Part model, mm, in its own coordinate system. A direction names the side the tool comes from. Give positions to 0.01 mm unless a question says otherwise; leave off trailing zeros. Write each loop counter-clockwise with the first axis right and the second up, starting at its lowest first coordinate (ties: lowest second). Pieces come first, ordered by that corner, then holes. Notation, with made-up numbers: M 43,28 L 58,28 A28 cw 58,63 Z; hole C 78,49.5 d5. An arc over 180 degrees is marked long. Write item = value, one per line. Start each with the question number.
Autodesk Inventor part; units mm, degrees
ref_plane "YZ Plane" through (0, 0, 0) normal (1, 0, 0) x (0, 1, 0)
ref_plane "XZ Plane" through (0, 0, 0) normal (0, 1, 0) x (-1, 0, 0)
ref_plane "XY Plane" through (0, 0, 0) normal (0, 0, 1) x (1, 0, 0)
sketch "Sketch1" plane through (0, 0, 0) normal (1, 0, 0) x (0, 1, 0)
  line L0 (0, 280.159) -> (0, -280.159)
  line L1 (0, 15) -> (100, 15)
  line L2 (100, 15) -> (100, 15)
  line L3 (105, 20) -> (125, 20)
  line L4 (130, 15) -> (130, -15)
  line L5 (125, -20) -> (105, -20)
  line L6 (100, -15) -> (100, -15)
  line L7 (100, -15) -> (0, -15)
  line L8 (0, 15) -> (0, -15)
  line L9 (0, 0) -> (130, 0)
  arc A0 (128, -20) -> (130, -18) centre (128, -18) ccw
  arc A1 (125, -20) -> (130, -15) centre (125, -15) ccw
  arc A2 (130, 15) -> (125, 20) centre (125, 15) ccw
  arc A3 (105, 20) -> (100, 15) centre (105, 15) ccw
  arc A4 (100, -15) -> (105, -20) centre (105, -15) ccw
  line L10 (10, 15) -> (10, -15)
  point P0 (130, 20)
  point P1 (130, -20)
  point P2 (100, -20)
  dimension "d0" = 560.3179
  dimension "d1" = 40
  dimension "d2" = 30
  dimension "d3" = 30
  dimension "d4" = 260
  dimension "d5" = 2
  dimension "d6" = 5
  dimension "d7" = 20
revolve "Revolution1" add sketch "Sketch1" angle 360 about axis through (0, 0, 280.159) along (0, 0, -1) contours L1 A3 L3 A2 L4 L9 L10 | L9 L4 A1 L5 A4 L7 L10
properties part number "wiel"
Q1. Slice it at C-C (z = -4.5). Give the cut face in (x, y), and give its area (3 significant figures).
Q2. Probe line 1 along X through (y, z) = (0, 8); line 2 along Z through (x, y) = (-35, -89); line 3 along Z through (x, y) = (-107, 65). List the from-to ranges inside material, lowest first.
Q3. Tool access for faces 1 (the face through (102, -28, -20)), 2 (the face through (-21, -1, 15)), 3 (the face through (-21, -1, -15)): list every direction of +Z, -Z, +X, -X, +Y, -Y with a clear straight run to the whole face (end or side of a thin tool).
Q4. Drop flat-ended pins along their axis: P1, Ø8, axis at x = 73, y = 0, coming from the +Z side; P2, Ø5, axis at x = 8.5, z = 7, coming from the -Y side; P3, Ø1, axis at y = 52, z = 9.5, coming from the -X side. Give the stop position or say it passes through.
Q5. Two-plate mould, pull along X, no slides. Class faces 4 (the face through (-9.76, -2.17, -0.21)), 5 (the face through (39.048, 123.997, -0.21)), 6 (the face through (102, -28, 20)): +X half, -X half, draft (parallel to the pull), parting line (faces both ways), or undercut.
Q6. Slice it at A-A (y = 0). Give the cut face in (x, z), and give its area (3 significant figures).
Working result:
q1.outline = C 0,0 d260; hole C 0,0 d20
q1.area = 52,800 mm2
q2.line_1 = -130 to -10, 10 to 130
q2.line_2 = -15 to 15
q2.line_3 = -20 to 20
q3.face_1 = -Z, +X, -X, +Y, -Y
q3.face_2 = +Z
q3.face_3 = -Z
q4.P1 = 15
q4.P2 = -129.86
q4.P3 = -119.36
q5.face_4 = undercut
q5.face_5 = parting line
q5.face_6 = draft
q6.outline = M -130,-15 A5 ccw -125,-20 L -105,-20 A5 ccw -100,-15 L -10,-15 L -10,15 L -100,15 A5 ccw -105,20 L -125,20 A5 ccw -130,15 Z; M 10,-15 L 100,-15 A5 ccw 105,-20 L 125,-20 A5 ccw 130,-15 L 130,15 A5 ccw 125,20 L 105,20 A5 ccw 100,15 L 10,15 Z
q6.area = 7,760 mm2
